Geometry: final body of the model. Coordinates: model frame, mm. Face numbers are marked on the shaded views. A direction names the side the tool comes from. Round coordinates to 2 decimals unless told otherwise and drop trailing zeros. Loops run counter-clockwise (first coordinate to the right, second up) from the corner with the lowest first, then second, coordinate; pieces in that order, holes last. Notation, with made-up numbers: (-8.75, 18) - (47.25, 18) arc R24 cw to (47.25, 37) - close; hole circle Ø7 at (52.25, -24). An arc over 180 degrees is marked (long way). Return JSON: item names as keys, results as strings. Group by question number.
1. Draft query along Y for the marked faces 1, 2, 3 and 4. Return one class per face: +Y half, -Y half, draft (parallel to the pull), parting line (faces both ways), or undercut.
2. Material intervals for probe 1 along Y at (x, z) = (-1, 2.25); probe 2 along Y at (x, z) = (-8, 4.25); probe 3 along X at (y, z) = (-3, 6), sorted ascending.
3. First-contact query: pin 1 Ø2 at (x, z) = (-11, 18) entering from -Y; pin 2 Ø3 at (x, y) = (-14, 2) entering from -Z. Flat tips, straight axial feed; report the tip coordinate or a pass-through.
4. Section A-A on x = -5. Return loops of the section in (y, z), and give its area (3 significant figures).
5. Set-up query: the marked faces 5, 6 and 7. Return all of +Z, -Z, +X, -X, +Y, -Y with unobstructed straight access to the full face (end or side cutting, diameter ignored); none if empty.
6. Section C-C on z = 10.5. Return loops of the section in (x, y).
7. Section B-B on y = 12.5. Return loops of the section in (x, z), and give its area (3 significant figures).
from build123d import *

# Parameters (mm, degrees)
F0_W        = 19.2
F0_H        = 100
F1_DEPTH    = 19.2
F2_W        = 15.4
F2_H        = 15.4
F3_DEPTH    = 18
F4_W        = 20
F4_H        = 10.5
F5_DEPTH    = 3
F6_T1_DEPTH = 29.25
F7_R        = 3.4
F8_DEPTH    = 25
F9_SIZE     = 0.5
F11_W       = 15.4
F11_H       = 15.4
F12_DEPTH   = 18


# Not quite as in the source:
# - a fillet or chamfer that OpenCascade refuses, or shapes differently, is made with other operations: its cross-section is extruded or revolved along the edge and cut away or added
# - a pattern or mirror of a feature is missing from the dataset's text; its kind, count and spacing are read off the source's solid


with BuildPart() as f1:
    # F0 (on Top) → F1 (new body)
    with BuildSketch(Plane.XY):
        Rectangle(F0_W, F0_H)
    extrude(amount=F1_DEPTH)

    # F2 (on face) → F3 (cut)
    with BuildSketch(Plane.YZ.offset(9.6)):
        with Locations((-40.4, 9.6)):
            Rectangle(F2_W, F2_H)
    f3 = extrude(amount=-F3_DEPTH, mode=Mode.SUBTRACT)

    # F3_copies: F3 across plane
    add(f3.mirror(Plane.ZX), mode=Mode.SUBTRACT)

    # F4 (on face) → F5 (join)
    with BuildSketch(Plane.XY.offset(19.2)):
        with Locations((-9.6, 0)):
            Rectangle(F4_W, F4_H)
    extrude(amount=-F5_DEPTH)

    # F6: fillet of radius 5.25 on 2 edges, made by hand

    # F6_s2 → F6_t1 (cut)
    with BuildSketch(Plane.XY.offset(3.075)):
        with BuildLine():
            ThreePointArc((-14.35, 5.25), (-18.0623106012, 3.7123106012), (-19.6, 0))
            Line((-19.6, 0), (-19.6, 5.25))
            Line((-19.6, 5.25), (-14.35, 5.25))
        make_face()
        with BuildLine():
            ThreePointArc((-14.35, -5.25), (-18.0623106012, -3.7123106012), (-19.6, 0))
            Line((-19.6, 0), (-19.6, -5.25))
            Line((-19.6, -5.25), (-14.35, -5.25))
        make_face()
    extrude(amount=F6_T1_DEPTH, mode=Mode.SUBTRACT)

    # F7 (on face) → F8 (cut)
    with BuildSketch(Plane.XY.offset(19.2)):
        with Locations((-14.35, 0)):
            Circle(F7_R)
    extrude(amount=-F8_DEPTH, mode=Mode.SUBTRACT)

    # F9
    f9_edges = [f1.edges().sort_by_distance(p)[0] for p in [
        (-9.6, 0, 0),
        (-9.6, -50, 9.6),
        (-9.6, -27.625, 19.2),
        (-9.6, -5.25, 17.7),
        (-9.6, 0, 16.2),
        (-9.6, 5.25, 17.7),
        (-9.6, 27.625, 19.2),
        (-9.6, 50, 9.6),
        (9.6, -50, 9.6),
        (0, -50, 0),
        (0, -50, 19.2),
        (9.6, 50, 9.6),
        (0, 50, 0),
        (0, 50, 19.2),
        (9.6, 0, 0),
        (9.6, 0, 19.2),
        (-11.975, -5.25, 19.2),
        (-18.062311, -3.712311, 19.2),
        (-18.062311, 3.712311, 19.2),
        (-11.975, 5.25, 19.2),
    ]]
    chamfer(f9_edges, length=F9_SIZE)

    # F11 (on face) → F12 (cut)
    with BuildSketch(Plane.XY.offset(19.2)):
        Rectangle(F11_W, F11_H)
    extrude(amount=-F12_DEPTH, mode=Mode.SUBTRACT)


solid = f1.part
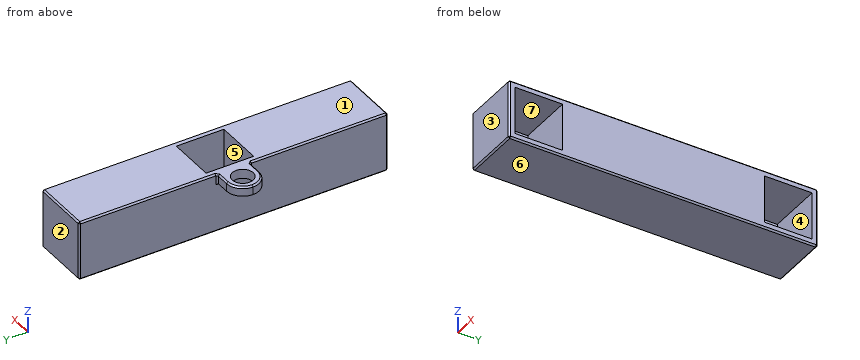
Taken from the geometry:
{
 "1": {"face 1": "draft", "face 2": "+Y half", "face 3": "-Y half", "face 4": "undercut"},
 "2": {"probe 1": "-50 to -48.1, -32.7 to -7.7, 7.7 to 32.7, 48.1 to 50", "probe 2": "-50 to -48.1, -32.7 to 32.7, 48.1 to 50", "probe 3": "-9.6 to -7.7, 7.7 to 9.6"},
 "3": {"pin 1": "y = -5.35", "pin 2": "z = 16.2"},
 "4": {"outline": "(-50, 0.5) - (-49.5, 0) - (49.5, 0) - (50, 0.5) - (50, 18.7) - (49.5, 19.2) - (7.7, 19.2) - (7.7, 1.2) - (-7.7, 1.2) - (-7.7, 19.2) - (-49.5, 19.2) - (-50, 18.7) - close; hole (-48.1, 1.9) - (-32.7, 1.9) - (-32.7, 17.3) - (-48.1, 17.3) - close; hole (32.7, 1.9) - (48.1, 1.9) - (48.1, 17.3) - (32.7, 17.3) - close", "area": "1,170 mm2"},
 "5": {"face 5": "+Z", "face 6": "-Z, +X, -X, +Y, -Y", "face 7": "+X"},
 "6": {"outline": "(-9.6, -49.5) - (-9.1, -50) - (9.1, -50) - (9.6, -49.5) - (9.6, -48.1) - (-8.4, -48.1) - (-8.4, -32.7) - (9.6, -32.7) - (9.6, 32.7) - (-8.4, 32.7) - (-8.4, 48.1) - (9.6, 48.1) - (9.6, 49.5) - (9.1, 50) - (-9.1, 50) - (-9.6, 49.5) - close; hole (-7.7, -7.7) - (7.7, -7.7) - (7.7, 7.7) - (-7.7, 7.7) - close"},
 "7": {"outline": "(-9.6, 0.5) - (-9.1, 0) - (9.1, 0) - (9.6, 0.5) - (9.6, 18.7) - (9.1, 19.2) - (-9.1, 19.2) - (-9.6, 18.7) - close", "area": "368 mm2"}
}
